Can you work these out from the model? Positions are in its coordinate system, mm. A direction names the side the tool comes from. Coordinates: 2 decimals unless noted, no trailing zeros. Order: outer loops, then holes, each group sorted by start corner. A loop starts at its lowest first (then second) coordinate and runs counter-clockwise, first axis right, second up. Notation, with made-up numbers: (34.25, 40) -> (40.25, 40) arc R17 cw to (40.25, 54) -> close; hole circle Ø6 at (46, 80). An arc over 180 degrees is marked (long way). Write item = value, one per line. Start each with the question number.
from build123d import *

# Parameters (mm, degrees)
BOSS_EXTRUDE1_DEPTH            = 50
HOLE_FOR_M5_300_SC_NUTS_SP_1_D = 10
HOLE_FOR_M5_300_SC_NUTS_SP_2_D = 3.5


with BuildPart() as part:
    # Sketch1 → Boss-Extrude1 (new body)
    with BuildSketch(Plane.XY):
        Polygon((-7.897485035, 31.347562808), (-7.897485035, 2.347562808), (14.102514965, 2.347562808), (14.102514965, -0.652437192), (-10.897485035, -0.652437192), (-10.897485035, 31.347562808), align=None)
    extrude(amount=BOSS_EXTRUDE1_DEPTH)

    # Hole for M5 300® SC Nuts (SP)1 (through all)
    with Locations(Plane(origin=(-7.897485035, 0, 0), x_dir=(0, 0, -1), z_dir=(1, 0, 0))):
        with Locations((-25, 22.347562808)):
            Hole(HOLE_FOR_M5_300_SC_NUTS_SP_1_D / 2)

    # Hole for M5 300® SC Nuts (SP)2 (through all)
    with Locations(Plane(origin=(-7.897485035, 0, 0), x_dir=(0, 0, -1), z_dir=(1, 0, 0))):
        with Locations((-17, 22.347562808), (-33, 22.347562808), (-25, 14.347562808)):
            Hole(HOLE_FOR_M5_300_SC_NUTS_SP_2_D / 2)


solid = part.part
(1) Imagine slicing it at A-A (z = 33). Write out the boundary of the cut face in (x, y), plus the area to 4 significant figures.
(2) Imagine slicing it at B-B (z = 25). Write out the boundary of the cut face in (x, y), plus the area to 4 significant figures.
(3) For faces 1 (the face through (14.103, 1, 25)), 2 (the face through (-7.897, 17, 25)), which set-ups out of +Z, -Z, +X, -X, +Y, -Y let a thin tool reach every point of the face, with its end or its side?
(4) For P1, Ø1.5, axis at y = 4, z = 20, coming from the +X side; P2, Ø3, axis at y = 14.35, z = 25, coming from the -X side; P3, Ø12, axis at y = 27, z = 23.5, coming from the -X side; P4, Ø11, axis at x = 4.5, z = 30, coming from the +Y side, each with a flat end and sliding along its axis, tell me the tip position at first contact or that it passes through.
(5) If I drill on L1, parallel to Y at x = -9.7, z = 33; L2, parallel to Y at x = -9.55, z = 25; L3, parallel to Y at x = 2.25, z = 36, over which ranges is the centre line in solid material (lowest first)? Write a range as from..to.
(6) Imagine slicing it at D-D (x = -6.75). Write out the boundary of the cut face in (y, z).
(7) Thinking about a two-plate mould opening in Y: for faces 3 (the face through (-9.4, 13.3, 23.6)), 4 (the face through (-9, 31.348, 25)), 5 (the face through (-9, 9, 50)), which applies, +Y half, -Y half, draft (parallel to the pull), parting line (faces both ways), or undercut?
(8) Imagine slicing it at C-C (y = 13.5). Write out the boundary of the cut face in (x, z), plus the area to 3 significant figures.
Result set:
q1.outline = (-10.9, -0.65) -> (14.1, -0.65) -> (14.1, 2.35) -> (-7.9, 2.35) -> (-7.9, 20.6) -> (-10.9, 20.6) -> close; (-10.9, 24.1) -> (-7.9, 24.1) -> (-7.9, 31.35) -> (-10.9, 31.35) -> close
q1.area = 151.5 mm2
q2.outline = (-10.9, -0.65) -> (14.1, -0.65) -> (14.1, 2.35) -> (-7.9, 2.35) -> (-7.9, 12.6) -> (-10.9, 12.6) -> close; (-10.9, 16.1) -> (-7.9, 16.1) -> (-7.9, 17.35) -> (-10.9, 17.35) -> close; (-10.9, 27.35) -> (-7.9, 27.35) -> (-7.9, 31.35) -> (-10.9, 31.35) -> close
q2.area = 121.5 mm2
q3.face_1 = +Z, -Z, +X, +Y, -Y
q3.face_2 = +Z, -Z, +X, +Y
q4.P1 = -7.9
q4.P2 = through
q4.P3 = -10.9
q4.P4 = 2.35
q5.L1 = -0.65..20.6, 24.1..31.35
q5.L2 = -0.65..12.6, 16.1..17.35, 27.35..31.35
q5.L3 = -0.65..2.35
q6.outline = (-0.65, 0) -> (2.35, 0) -> (2.35, 50) -> (-0.65, 50) -> close
q7.face_3 = undercut
q7.face_4 = +Y half
q7.face_5 = draft
q8.outline = (-10.9, 0) -> (-7.9, 0) -> (-7.9, 23.47) -> (-10.9, 23.47) -> close; (-10.9, 26.53) -> (-7.9, 26.53) -> (-7.9, 50) -> (-10.9, 50) -> close
q8.area = 141 mm2
